Read the model definition and answer for the solid it produces. Units are mm, in the model's axes. Face numbers are marked on the shaded views. Coordinates: 2 decimals unless noted, no trailing zeros. Loops run counter-clockwise (first coordinate to the right, second up) from the corner with the lowest first, then second, coordinate; pieces in that order, holes last. Notation, with made-up numbers: (83.5, -2) -> (130.5, -2) arc R27 ccw to (130.5, 18) -> close; hole circle Ø10 at (52.5, 68). An arc over 180 degrees is marked (long way). Answer as a JSON object with one key per item and string values. Group by question number.
Q1. Determine the mould class of the marked faces 1, 2, 3 and 4 for opening direction X: released by +X, released by -X, zero draft, split by the parting line, or undercut.
Q2. The part is cut by section C-C on z = 3.5. Write down the section's boundary in (x, y), and give its area (3 significant figures).
Q3. The part is cut by section B-B on y = 0. Write down the section's boundary in (x, z), and give its area (3 significant figures).
Q4. Straight lines are drawn through the part: line 1 along Y through (x, z) = (19, 2.25); line 2 along X through (y, z) = (0.25, 5); line 3 along Y through (x, z) = (-19, 3.75). For each, find the intervals that lie inside material, in ascending order. Write a range as [from, to].
Q5. The part is cut by section D-D on x = 19. Write down the section's boundary in (y, z).
Q6. The part is cut by section A-A on x = -19. Write down the section's boundary in (y, z), and give its area (3 significant figures).
Q7. This flat-tipped pin is pushed along its axis until it touches: P1, Ø1.5, axis at x = -15.5, y = 0, coming from the +Z side. Where does it stop, or does it pass through?
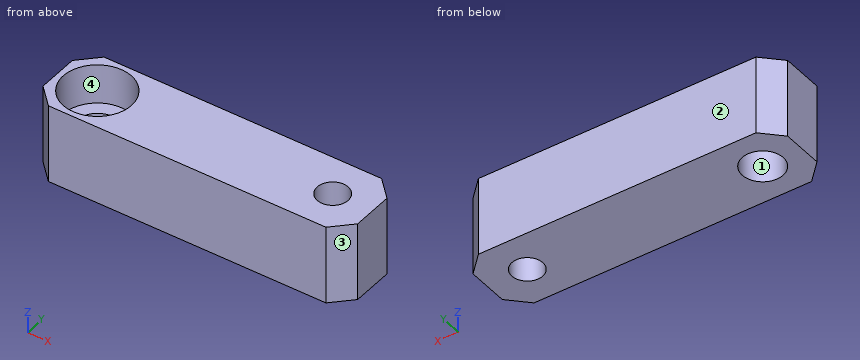
from build123d import *

# Parameters (mm, degrees)
SALIENTE_EXTRUIR1_DEPTH                              = 6.35
TALADRO_ROSCADO_M61_D                                = 5
REFRENTADO_PARA_TORNILLO_CON_CABEZA_HUEC_D           = 6.6
REFRENTADO_PARA_TORNILLO_CON_CABEZA_HUEC_CBORE_D     = 11
REFRENTADO_PARA_TORNILLO_CON_CABEZA_HUEC_CBORE_DEPTH = 6.4


with BuildPart() as part:
    # Croquis1 → Saliente-Extruir1 (new, symmetric)
    with BuildSketch(Plane.XY):
        Polygon((-22.4, 6.35), (-25.4, 3.35), (-25.4, -3.35), (-22.4, -6.35), (22.4, -6.35), (25.4, -3.35), (25.4, 3.35), (22.4, 6.35), align=None)
    extrude(amount=SALIENTE_EXTRUIR1_DEPTH, both=True)

    # Taladro roscado M61 (through all)
    with Locations(Plane.XY.offset(6.35)):
        with Locations((19, 0)):
            Hole(TALADRO_ROSCADO_M61_D / 2)

    # Refrentado para tornillo con cabeza huec (through all)
    with Locations(Plane.XY.offset(6.35)):
        with Locations((-19, 0)):
            CounterBoreHole(REFRENTADO_PARA_TORNILLO_CON_CABEZA_HUEC_D / 2, REFRENTADO_PARA_TORNILLO_CON_CABEZA_HUEC_CBORE_D / 2, REFRENTADO_PARA_TORNILLO_CON_CABEZA_HUEC_CBORE_DEPTH)


solid = part.part
Final values:
{
 "1": {"face 1": "undercut", "face 2": "zero draft", "face 3": "released by +X", "face 4": "undercut"},
 "2": {"outline": "(-25.4, -3.35) -> (-22.4, -6.35) -> (22.4, -6.35) -> (25.4, -3.35) -> (25.4, 3.35) -> (22.4, 6.35) -> (-22.4, 6.35) -> (-25.4, 3.35) -> close; hole circle Ø11 at (-19, 0); hole circle Ø5 at (19, 0)", "area": "512 mm2"},
 "3": {"outline": "(-25.4, -6.35) -> (-22.3, -6.35) -> (-22.3, -0.05) -> (-24.5, -0.05) -> (-24.5, 6.35) -> (-25.4, 6.35) -> close; (-15.7, -6.35) -> (16.5, -6.35) -> (16.5, 6.35) -> (-13.5, 6.35) -> (-13.5, -0.05) -> (-15.7, -0.05) -> close; (21.5, -6.35) -> (25.4, -6.35) -> (25.4, 6.35) -> (21.5, 6.35) -> close", "area": "470 mm2"},
 "4": {"line 1": "y = [-6.35, -2.5], [2.5, 6.35]", "line 2": "x = [-25.4, -24.49], [-13.51, 16.51], [21.49, 25.4]", "line 3": "y = [-6.35, -5.5], [5.5, 6.35]"},
 "5": {"outline": "(-6.35, -6.35) -> (-2.5, -6.35) -> (-2.5, 6.35) -> (-6.35, 6.35) -> close; (2.5, -6.35) -> (6.35, -6.35) -> (6.35, 6.35) -> (2.5, 6.35) -> close"},
 "6": {"outline": "(-6.35, -6.35) -> (-3.3, -6.35) -> (-3.3, -0.05) -> (-5.5, -0.05) -> (-5.5, 6.35) -> (-6.35, 6.35) -> close; (3.3, -6.35) -> (6.35, -6.35) -> (6.35, 6.35) -> (5.5, 6.35) -> (5.5, -0.05) -> (3.3, -0.05) -> close", "area": "49.3 mm2"},
 "7": {"P1": "stops at z = -0.05"}
}
